Input: dimensioned drawing with shaded views. Units: mm. Origin: part minimum x, y, z. Round coordinates to 2 decimals unless told otherwise and drop trailing zeros. Order: outer loops, then holes, each group sorted by start corner. A loop starts at its lowest first (then second) coordinate and runs counter-clockwise, first axis right, second up. Notation, with made-up numbers: (-5.75, 25) - (20.25, 25) arc R27 ccw to (20.25, 58) - close; hole circle Ø11 at (72.25, 5.5). An arc over 180 degrees is marked (long way). Return JSON: item names as keys, results as strings. Group by question number.
1) Ray query, line 1 (X direction, y = 5.5, z = 15); line 2 (Z direction, x = 75, y = 7.75); line 3 (X direction, y = 4.75, z = 17.5). Return the intervals inside material, ascending. Write a range as from..to.
2) Contact query for a flat-ended pin moving along its axis: P1, Ø3.5, axis at x = 25, z = 15, coming from the +Y side. Output: stop coordinate, or through.
3) Section A-A, the plane z = 15. Return loops of the section in (x, y).
4) Section B-B, the plane x = 25. Return loops of the section in (y, z), plus the area to 3 significant figures.
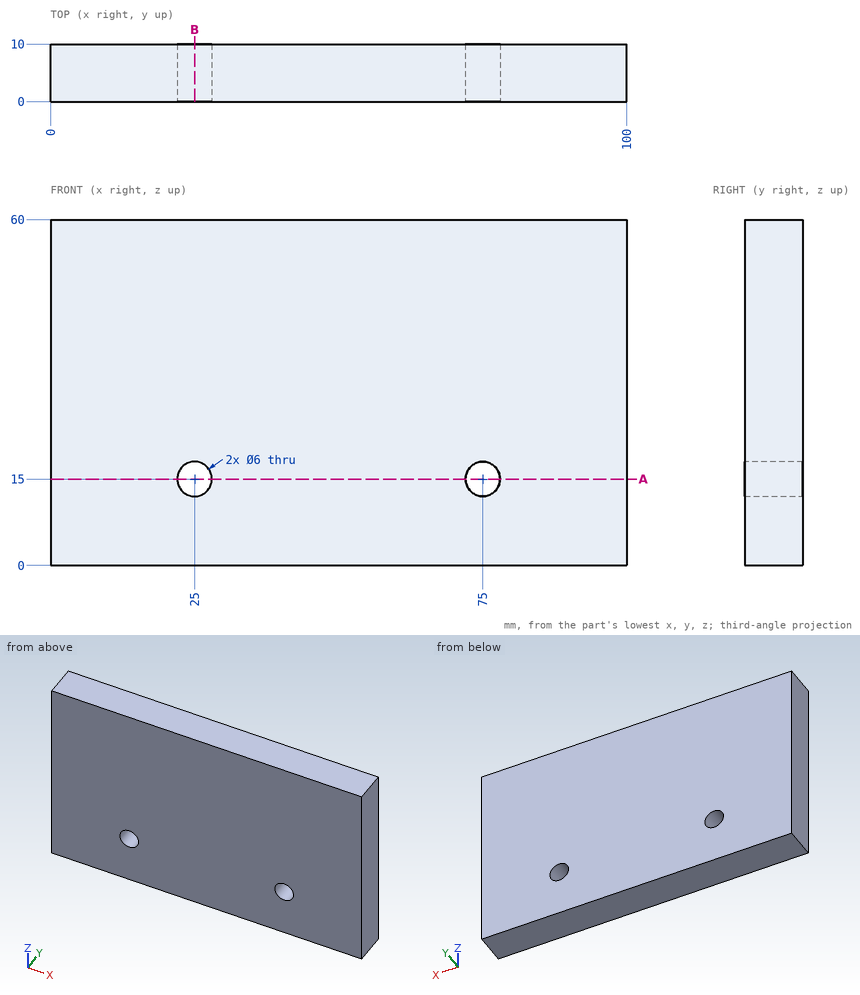
Geometry check:
{
 "1": {"line 1": "0..22, 28..72, 78..100", "line 2": "0..12, 18..60", "line 3": "0..23.34, 26.66..73.34, 76.66..100"},
 "2": {"P1": "through"},
 "3": {"outline": "(0, 0) - (22, 0) - (22, 10) - (0, 10) - close; (28, 0) - (72, 0) - (72, 10) - (28, 10) - close; (78, 0) - (100, 0) - (100, 10) - (78, 10) - close"},
 "4": {"outline": "(0, 0) - (10, 0) - (10, 12) - (0, 12) - close; (0, 18) - (10, 18) - (10, 60) - (0, 60) - close", "area": "540 mm2"}
}
